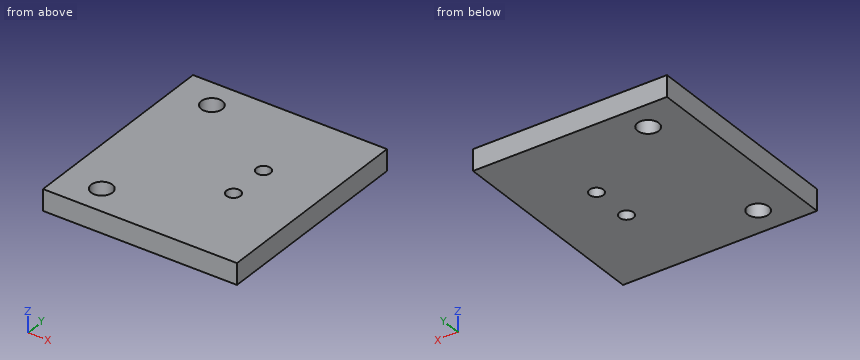
from build123d import *

# Parameters (mm, degrees)
CROQUIS1_W              = 27.5
CROQUIS1_H              = 30
CROQUIS1_R              = 1
CROQUIS1_R_2            = 1.5
SALIENTE_EXTRUIR1_DEPTH = 3


with BuildPart() as part:
    # Croquis1 → Saliente-Extruir1 (new body)
    with BuildSketch(Plane.XY):
        with Locations((13.75, 15)):
            Rectangle(CROQUIS1_W, CROQUIS1_H)
        with Locations((18.5, 12)):
            Circle(CROQUIS1_R, mode=Mode.SUBTRACT)
        with Locations((18.5, 18)):
            Circle(CROQUIS1_R, mode=Mode.SUBTRACT)
        with Locations((5.5, 4)):
            Circle(CROQUIS1_R_2, mode=Mode.SUBTRACT)
        with Locations(Location((5.5, 26, 0), (0, 0, 180))):
            Circle(CROQUIS1_R_2, mode=Mode.SUBTRACT)
    extrude(amount=SALIENTE_EXTRUIR1_DEPTH)


solid = part.part
Here's how the part is built. I have some questions about the finished solid (model axes, mm). Round coordinates to 2 decimals unless told otherwise and drop trailing zeros. Write each loop counter-clockwise with the first axis right and the second up, starting at its lowest first coordinate (ties: lowest second). Pieces come first, ordered by that corner, then holes. Notation, with made-up numbers: (56.5, 84) -> (107.5, 84) arc R12 cw to (107.5, 89) -> close; hole circle Ø2 at (45.25, 77.5). An arc over 180 degrees is marked (long way). One line per item, written item: value.
1) Suppose I cut it at C-C on x = 18.5. List the corners of the cut face in (y, z) for me.
Filled sheet:
outline: (0, 0) -> (11, 0) -> (11, 3) -> (0, 3) -> close; (13, 0) -> (17, 0) -> (17, 3) -> (13, 3) -> close; (19, 0) -> (30, 0) -> (30, 3) -> (19, 3) -> close
2) If I drill on line 1 (Y direction, x = 5.5, z = 2.3); line 2 (X direction, y = 17.5, z = 1.15); line 3 (Y direction, x = 6.5, z = 0.2), over which ranges is the centre line in solid material (lowest first)? Write a range as [from, to].
Filled sheet:
line 1: y = [0, 2.5], [5.5, 24.5], [27.5, 30]
line 2: x = [0, 17.63], [19.37, 27.5]
line 3: y = [0, 2.88], [5.12, 24.88], [27.12, 30]
3) Suppose I cut it at D-D on y = 26. List the corners of the cut face in (x, z) for me.
Filled sheet:
outline: (0, 0) -> (4, 0) -> (4, 3) -> (0, 3) -> close; (7, 0) -> (27.5, 0) -> (27.5, 3) -> (7, 3) -> close
4) Suppose I cut it at A-A on y = 12. List the corners of the cut face in (x, z) for me, plus the area to 3 significant figures.
Filled sheet:
outline: (0, 0) -> (17.5, 0) -> (17.5, 3) -> (0, 3) -> close; (19.5, 0) -> (27.5, 0) -> (27.5, 3) -> (19.5, 3) -> close
area: 76.5 mm2
5) I'm going to push a flat-ended pin straight in: pin 1 Ø1.6 at (x, y) = (18.5, 12) entering from -Z (1 decimal). Where does the tip first touch, or does it pass through?
Filled sheet:
pin 1: passes through
6) Suppose I cut it at B-B on z = 2.55. List the corners of the cut face in (x, y) for me, plus the area to 3 significant figures.
Filled sheet:
outline: (0, 0) -> (27.5, 0) -> (27.5, 30) -> (0, 30) -> close; hole circle Ø3 at (5.5, 4); hole circle Ø3 at (5.5, 26); hole circle Ø2 at (18.5, 12); hole circle Ø2 at (18.5, 18)
area: 805 mm2
